```python
from build123d import *

# Parameters (mm, degrees)
BOSS_EXTRUDE1_DEPTH   = 254
M3_CLEARANCE_HOLE1_D  = 3.4
F_8_CLEARANCE_HOLE1_D = 4.4958


with BuildPart() as part:
    # Sketch1 → Boss-Extrude1 (new body)
    with BuildSketch(Plane(origin=(0, 0, 0), x_dir=(0, 0, -1), z_dir=(1, 0, 0))):
        Polygon((0, 0), (-34.925, 0), (-34.925, -3.175), (3.175, -3.175), (3.175, 34.925), (0, 34.925), align=None)
    extrude(amount=BOSS_EXTRUDE1_DEPTH)

    # M3 Clearance Hole1 (through all)
    with Locations(Plane.XY):
        with Locations((17, 30.825), (17, 10.825), (237, 10.825), (237, 30.825)):
            Hole(M3_CLEARANCE_HOLE1_D / 2)

    # #8 Clearance Hole1 (through all)
    with Locations(Plane(origin=(0, 0, 0), x_dir=(1, 0, 0), z_dir=(0, 1, 0))):
        with Locations((25.4, -15.875), (228.6, -15.875)):
            Hole(F_8_CLEARANCE_HOLE1_D / 2)


solid = part.part
```
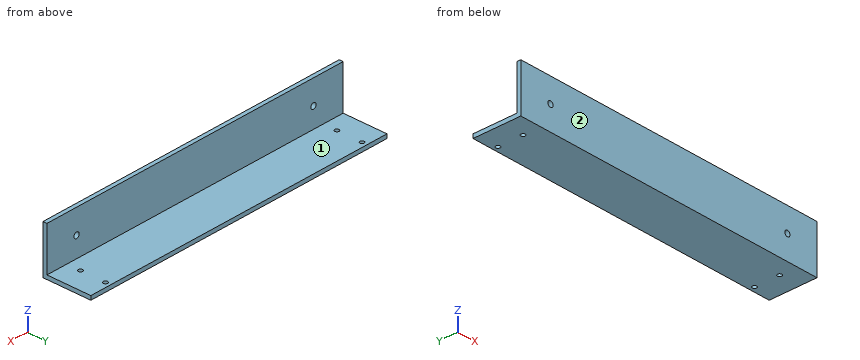
Input: part model. Units: mm. Frame: model coordinates. Face numbers are marked on the shaded views. A direction names the side the tool comes from. Coordinates: 2 decimals unless noted, no trailing zeros. Loops run counter-clockwise (first coordinate to the right, second up) from the corner with the lowest first, then second, coordinate; pieces in that order, holes last.
Q1. Set-up query: the marked faces 1 and 2. Return all of +Z, -Z, +X, -X, +Y, -Y with unobstructed straight access to the full face (end or side cutting, diameter ignored); none if empty.
Results are:
face 1: +Z, +X, -X, +Y
face 2: +Z, -Z, +X, -X, -Y
Q2. Section C-C, the plane z = 10.5. Return the cut outline in (x, y) (3 decimals).
Results are:
outline: (0, -3.175) - (254, -3.175) - (254, 0) - (0, 0) - close
Q3. Section A-A, the plane x = 228.6. Return the cut outline in (y, z) (3 decimals), and give its area (3 significant figures).
Results are:
outline: (-3.175, -3.175) - (34.925, -3.175) - (34.925, 0) - (0, 0) - (0, 13.627) - (-3.175, 13.627) - close; (-3.175, 18.123) - (0, 18.123) - (0, 34.925) - (-3.175, 34.925) - close
area: 218 mm2
Q4. Section B-B, the plane x = 112.5. Return the cut outline in (y, z) (3 decimals).
Results are:
outline: (-3.175, -3.175) - (34.925, -3.175) - (34.925, 0) - (0, 0) - (0, 34.925) - (-3.175, 34.925) - close
Q5. Contact query for flat-ended pins moving along their axis: pin 1 (2 mm diameter, centred on x = 200, y = 13, fed in from +Z); pin 2 (4 mm diameter, centred on x = 237, y = 10.825, fed in from -Z) (3 decimals); pin 3 (8 mm diameter, centred on x = 124.5, z = 31, fed in from +Y); pin 4 (3 mm diameter, centred on x = 237, y = 30.825, fed in from +Z). Output: stop coordinate, or through.
Results are:
pin 1: stops at z = 0
pin 2: stops at z = -3.175
pin 3: stops at y = 0
pin 4: passes through
Q6. Line query: line 1 along Y through (x, z) = (17, -1.6) (3 decimals); line 2 along Z through (x, y) = (228.6, -0.75) (3 decimals); line 3 along Z through (x, y) = (22, 19) (3 decimals). Output: solid intervals per line, ascending.
Results are:
line 1: y = -3.175 to 9.125, 12.525 to 29.125, 32.525 to 34.925
line 2: z = -3.175 to 13.627, 18.123 to 34.925
line 3: z = -3.175 to 0
